```python
from build123d import *

# Parameters (mm, degrees)
CROQUIS1_W                = 69.2
CROQUIS1_H                = 86
CROQUIS1_R                = 22.5
CROQUIS1_R_2              = 2.75
SALIENTE_EXTRUIR1_DEPTH   = 5
CROQUIS8_R                = 4
CORTAR_EXTRUIR3_DEPTH     = 5
TALADRO_ROSCADO_M42_D     = 3.3
TALADRO_ROSCADO_M62_D     = 5
TALADRO_ROSCADO_M62_DEPTH = 18
TALADRO_ROSCADO_M62_TIP   = 1.502151548
TALADRO_ROSCADO_M63_D     = 5
TALADRO_ROSCADO_M63_DEPTH = 18
TALADRO_ROSCADO_M63_TIP   = 1.502151548
CROQUIS15_R               = 37.5
CORTAR_EXTRUIR4_DEPTH     = 1


with BuildPart() as part:
    # Croquis1 → Saliente-Extruir1 (new body, symmetric)
    with BuildSketch(Plane.XY):
        with Locations((0.4, 0)):
            Rectangle(CROQUIS1_W, CROQUIS1_H)
        Circle(CROQUIS1_R, mode=Mode.SUBTRACT)
        with Locations((0, 34.3)):
            Circle(CROQUIS1_R_2, mode=Mode.SUBTRACT)
        with Locations((29.70467135, 17.15)):
            Circle(CROQUIS1_R_2, mode=Mode.SUBTRACT)
        with Locations((29.70467135, -17.15)):
            Circle(CROQUIS1_R_2, mode=Mode.SUBTRACT)
        with Locations((0, -34.3)):
            Circle(CROQUIS1_R_2, mode=Mode.SUBTRACT)
        with Locations((-29.70467135, -17.15)):
            Circle(CROQUIS1_R_2, mode=Mode.SUBTRACT)
        with Locations((-29.70467135, 17.15)):
            Circle(CROQUIS1_R_2, mode=Mode.SUBTRACT)
    extrude(amount=SALIENTE_EXTRUIR1_DEPTH, both=True)

    # Croquis8 → Cortar-Extruir3 (cut)
    with BuildSketch(Plane.XY.offset(5)):
        with Locations((-29.70467135, 17.15)):
            Circle(CROQUIS8_R)
        with Locations((0, 34.3)):
            Circle(CROQUIS8_R)
        with Locations((29.70467135, 17.15)):
            Circle(CROQUIS8_R)
        with Locations((29.70467135, -17.15)):
            Circle(CROQUIS8_R)
        with Locations((0, -34.3)):
            Circle(CROQUIS8_R)
        with Locations((-29.70467135, -17.15)):
            Circle(CROQUIS8_R)
    extrude(amount=-CORTAR_EXTRUIR3_DEPTH, mode=Mode.SUBTRACT)

    # Taladro roscado M42 (through all)
    with Locations(Plane.XY.offset(5)):
        with Locations((-12.5, 21.650635095), (-12.5, -21.650635095), (25, 0)):
            Hole(TALADRO_ROSCADO_M42_D / 2)

    # Taladro roscado M62
    with Locations(Plane(origin=(0, 43, 0), x_dir=(-1, 0, 0), z_dir=(0, 1, 0))):
        with Locations((25, -0.5), (-25, -0.5)):
            Hole(TALADRO_ROSCADO_M62_D / 2, depth=TALADRO_ROSCADO_M62_DEPTH)
            with Locations((0, 0, -(TALADRO_ROSCADO_M62_DEPTH + TALADRO_ROSCADO_M62_TIP / 2))):  # 118° drill point
                Cone(0, TALADRO_ROSCADO_M62_D / 2, TALADRO_ROSCADO_M62_TIP, mode=Mode.SUBTRACT)

    # Taladro roscado M63
    with Locations(Plane.XZ.offset(43)):
        with Locations((-25, -0.5), (25, -0.5)):
            Hole(TALADRO_ROSCADO_M63_D / 2, depth=TALADRO_ROSCADO_M63_DEPTH)
            with Locations((0, 0, -(TALADRO_ROSCADO_M63_DEPTH + TALADRO_ROSCADO_M63_TIP / 2))):  # 118° drill point
                Cone(0, TALADRO_ROSCADO_M63_D / 2, TALADRO_ROSCADO_M63_TIP, mode=Mode.SUBTRACT)

    # Croquis15 → Cortar-Extruir4 (cut)
    with BuildSketch(Plane(origin=(0, 0, -5), x_dir=(-1, 0, 0), z_dir=(0, 0, -1))):
        Circle(CROQUIS15_R)
    extrude(amount=-CORTAR_EXTRUIR4_DEPTH, mode=Mode.SUBTRACT)


solid = part.part
```
Read the model definition and answer for the solid it produces. Units are mm, in the model's axes. A direction names the side the tool comes from. Coordinates: 2 decimals unless noted, no trailing zeros. Write each loop counter-clockwise with the first axis right and the second up, starting at its lowest first coordinate (ties: lowest second). Pieces come first, ordered by that corner, then holes. Notation, with made-up numbers: (-3, -1) -> (18, -1) arc R11 ccw to (18, 16) -> close; hole circle Ø3 at (10.25, 51). An arc over 180 degrees is marked (long way). Write item = value, one per line.
(1) Section B-B on y = -34.3 is taken. Write down the section's boundary in (x, z).
From the geometry:
outline = (-34.2, -5) -> (-15.16, -5) -> (-15.16, -4) -> (-2.75, -4) -> (-2.75, 0) -> (-4, 0) -> (-4, 5) -> (-34.2, 5) -> close; (2.75, -4) -> (15.16, -4) -> (15.16, -5) -> (35, -5) -> (35, 5) -> (4, 5) -> (4, 0) -> (2.75, 0) -> close; hole circle Ø5 at (-25, -0.5); hole circle Ø5 at (25, -0.5)
(2) Section A-A on x = 0 is taken. Write down the section's boundary in (y, z).
From the geometry:
outline = (-43, -5) -> (-37.5, -5) -> (-37.5, -4) -> (-37.05, -4) -> (-37.05, 0) -> (-38.3, 0) -> (-38.3, 5) -> (-43, 5) -> close; (-31.55, -4) -> (-22.5, -4) -> (-22.5, 5) -> (-30.3, 5) -> (-30.3, 0) -> (-31.55, 0) -> close; (22.5, -4) -> (31.55, -4) -> (31.55, 0) -> (30.3, 0) -> (30.3, 5) -> (22.5, 5) -> close; (37.05, -4) -> (37.5, -4) -> (37.5, -5) -> (43, -5) -> (43, 5) -> (38.3, 5) -> (38.3, 0) -> (37.05, 0) -> close
(3) Straight lines are drawn through the part: L1, parallel to X at y = -36.5, z = -0.5; L2, parallel to Y at x = 0, z = -3.15; L3, parallel to Y at x = 0, z = 3.25. For each, find the intervals that lie inside material, in ascending order. Write a range as from..to.
From the geometry:
L1 = -34.2..-27.5, -22.5..-1.65, 1.65..22.5, 27.5..35
L2 = -43..-37.05, -31.55..-22.5, 22.5..31.55, 37.05..43
L3 = -43..-38.3, -30.3..-22.5, 22.5..30.3, 38.3..43
(4) Which of the six approach directions +Z, -Z, +X, -X, +Y, -Y give full straight-line access (tool end or side, diameter ignored) to faces 4 (the face through (10.382, -19.961, 0.437)), 5 (the face through (-29, 20, 0)), 6 (the face through (27.5, -33.9, -0.4))?
From the geometry:
face_4 = +Z, -Z
face_5 = +Z
face_6 = -Y
(5) Given pin 1 Ø4 at (x, z) = (-25, -0.5) entering from +Y; pin 2 Ø5 at (x, y) = (26.5, 2.5) entering from -Z; pin 3 Ø7 at (x, y) = (-29.7, 17.15) entering from +Z, each flat-ended and moving along its own axis, determine where each tip first touches the part or whether it passes through.
From the geometry:
pin_1 = 24.7
pin_2 = -4
pin_3 = 0
(6) Section C-C on x = -18 is taken. Write down the section's boundary in (y, z).
From the geometry:
outline = (-43, -5) -> (-32.9, -5) -> (-32.9, -4) -> (-13.5, -4) -> (-13.5, 5) -> (-43, 5) -> close; (13.5, -4) -> (32.9, -4) -> (32.9, -5) -> (43, -5) -> (43, 5) -> (13.5, 5) -> close
(7) For a pull along Z with two mould halves and no side action, classify faces 1 (the face through (29.109, -19.835, -2.028)), 2 (the face through (-25.4, 23.76, -0.67)), 3 (the face through (29, -20, 0)) as +Z half, -Z half, draft (parallel to the pull), parting line (faces both ways), or undercut.
From the geometry:
face_1 = draft
face_2 = undercut
face_3 = +Z half
(8) Section D-D on y = 0 is taken. Write down the section's boundary in (x, z), plus the area to 3 significant figures.
From the geometry:
outline = (-34.2, -4) -> (-22.5, -4) -> (-22.5, 5) -> (-34.2, 5) -> close; (22.5, -4) -> (23.35, -4) -> (23.35, 5) -> (22.5, 5) -> close; (26.65, -4) -> (35, -4) -> (35, 5) -> (26.65, 5) -> close
area = 188 mm2
